The drawing under review shows one solid part. Ordinate dimensions are in mm from its lowest x, y, z. Give positions to 0.01 mm unless a question says otherwise; leave off trailing zeros. Loops run counter-clockwise (first coordinate to the right, second up) from the corner with the lowest first, then second, coordinate; pieces in that order, holes last. Notation, with made-up numbers: M 65.5,-20.75 L 105.5,-20.75 A12 cw 105.5,-1.75 Z; hole C 54.25,17.5 d8. An arc over 180 degrees is marked long. Answer as CSV lines item,"result".
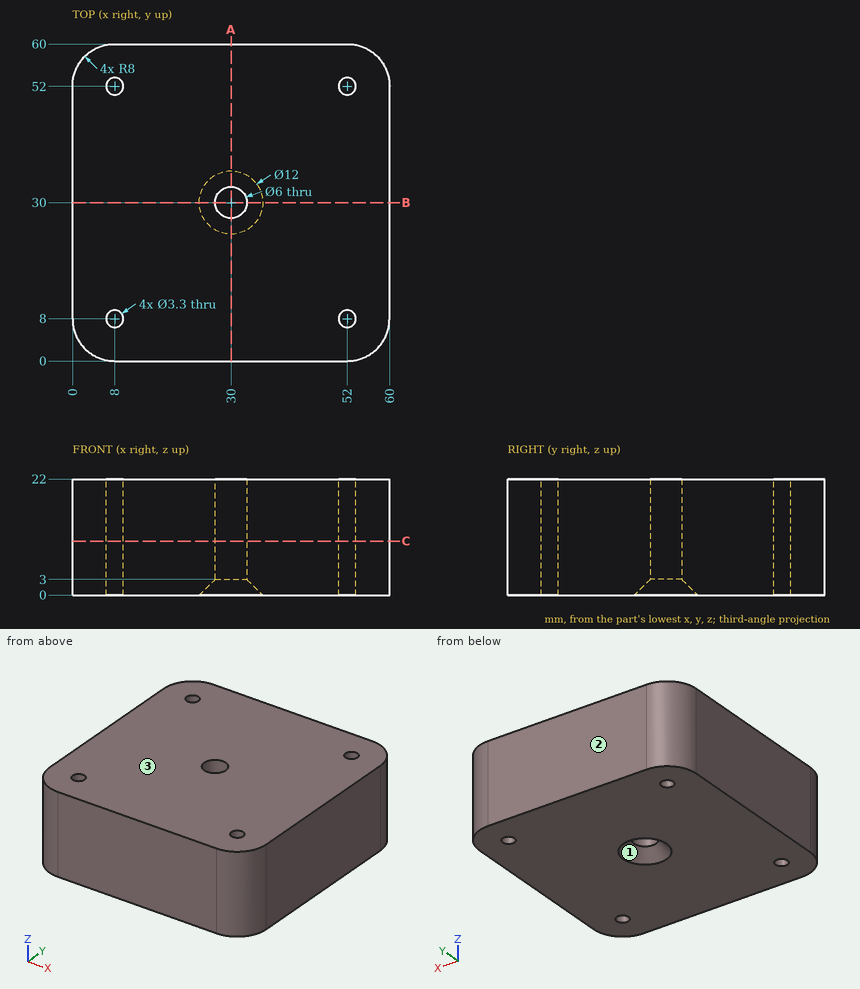
1. We need section A-A, the plane x = 30. Write out the cut boundary in (y, z), plus the area to 3 significant figures.
Answer block:
outline,"M 0,0 L 24,0 L 27,3 L 27,22 L 0,22 Z; M 33,3 L 36,0 L 60,0 L 60,22 L 33,22 Z"
area,"1,180 mm²"
2. For P1, Ø3, axis at x = 8, y = 52, coming from the +Z side, flat-tipped, find the tip position at first contact; note if it passes through.
Answer block:
P1,"through"
3. The part is to be moulded in two halves that separate along Y. For the marked faces 1, 2 and 3, say which applies: pulls with the +Y half, pulls with the -Y half, needs draft (parallel to the pull), parting line crosses it, or undercut.
Answer block:
face 1,"undercut"
face 2,"pulls with the +Y half"
face 3,"needs draft"
4. To check wall thickness, follow L1, parallel to Y at x = 52, z = 8.5; L2, parallel to X at y = 29, z = 11; L3, parallel to Y at x = 32.5, z = 19.75. State the ranges of each line that lie inside material, in increasing order. Write a range as [from, to].
Answer block:
L1,"[0, 6.35], [9.65, 50.35], [53.65, 60]"
L2,"[0, 27.17], [32.83, 60]"
L3,"[0, 28.34], [31.66, 60]"
5. We need section C-C, the plane z = 10.25. Write out the cut boundary in (x, y).
Answer block:
outline,"M 0,8 A8 ccw 8,0 L 52,0 A8 ccw 60,8 L 60,52 A8 ccw 52,60 L 8,60 A8 ccw 0,52 Z; hole C 8,8 d3.3; hole C 8,52 d3.3; hole C 30,30 d6; hole C 52,8 d3.3; hole C 52,52 d3.3"
